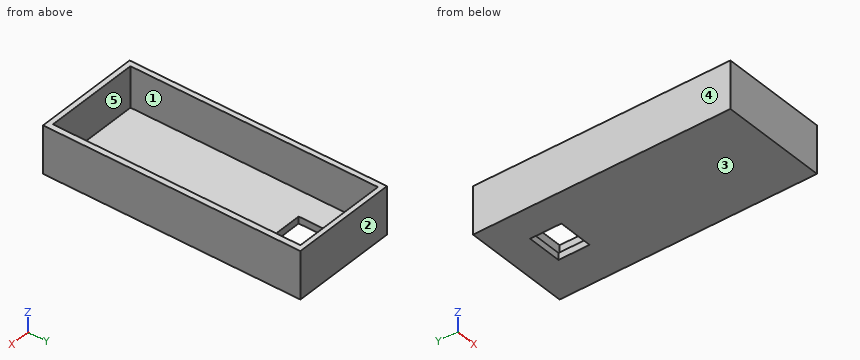
from build123d import *

# Parameters (mm, degrees)
F0_W     = 50
F0_H     = 120
F1_DEPTH = 22.1
F2_W     = 44.786031
F2_H     = 115.363243
F3_DEPTH = 18.9
F4_W     = 16.371712
F4_H     = 14.506579
F5_DEPTH = 3.2


with BuildPart() as f1:
    # F0 (on Top) → F1 (new body)
    with BuildSketch(Plane.XY):
        with Locations((25, 60)):
            Rectangle(F0_W, F0_H)
    extrude(amount=F1_DEPTH)

    # F2 (on face) → F3 (cut)
    with BuildSketch(Plane.XY.offset(22.1)):
        with Locations((24.874761, 60.085734)):
            Rectangle(F2_W, F2_H)
    extrude(amount=-F3_DEPTH, mode=Mode.SUBTRACT)

    # F4 (on face) → F5 (cut, through all)
    with BuildSketch(Plane.XY.offset(3.2)):
        with Locations((23.106907, 98.141447)):
            Rectangle(F4_W, F4_H)
    extrude(amount=-F5_DEPTH, mode=Mode.SUBTRACT)


solid = f1.part
Can you work these out from the model? Positions are in its coordinate system, mm. Face numbers are marked on the shaded views. A direction names the side the tool comes from. Round coordinates to 2 decimals unless told otherwise and drop trailing zeros. Write each loop counter-clockwise with the first axis right and the second up, starting at its lowest first coordinate (ties: lowest second). Pieces come first, ordered by that corner, then holes. Notation, with made-up numbers: M 86.5,84.25 L 144.5,84.25 A8 cw 144.5,96.25 Z; hole C 20,46.25 d11. An arc over 180 degrees is marked long. Use a Markdown table: item, result.
Item 1: Which directions (+Z, -Z, +X, -X, +Y, -Y) give clear straight access to the entire face, cutting with the end or side of a thin tool? Please do the marked faces 1 and 2.
Found:
| item | result |
|---|---|
| face 1 | +Z |
| face 2 | +Z, -Z, +X, -X, +Y |
Item 2: For pin 1 Ø2 at (x, y) = (35, 20.5) entering from +Z, with a flat end and sliding along its axis, tell me the tip position at first contact or that it passes through.
Found:
| item | result |
|---|---|
| pin 1 | stops at z = 3.2 |
Item 3: We'd pull the mould along X, two halves only. Please class the marked faces 3, 4 and 5: released by +X, released by -X, zero draft, split by the parting line, or undercut.
Found:
| item | result |
|---|---|
| face 3 | zero draft |
| face 4 | released by -X |
| face 5 | undercut |
Item 4: I want a section at C-C (y = 80). List the corners of the cut face in (x, z) for me.
Found:
| item | result |
|---|---|
| outline | M 0,0 L 50,0 L 50,22.1 L 47.27,22.1 L 47.27,3.2 L 2.48,3.2 L 2.48,22.1 L 0,22.1 Z |
Item 5: I want a section at D-D (x = 7). List the corners of the cut face in (y, z) for me, and give its area (3 significant figures).
Found:
| item | result |
|---|---|
| outline | M 0,0 L 120,0 L 120,22.1 L 117.77,22.1 L 117.77,3.2 L 2.4,3.2 L 2.4,22.1 L 0,22.1 Z |
| area | 472 mm2 |
Item 6: I want a section at A-A (x = 30). List the corners of the cut face in (y, z) for me.
Found:
| item | result |
|---|---|
| outline | M 0,0 L 90.89,0 L 90.89,3.2 L 2.4,3.2 L 2.4,22.1 L 0,22.1 Z; M 105.39,0 L 120,0 L 120,22.1 L 117.77,22.1 L 117.77,3.2 L 105.39,3.2 Z |
Item 7: I want a section at B-B (z = 15.25). List the corners of the cut face in (x, y) for me.
Found:
| item | result |
|---|---|
| outline | M 0,0 L 50,0 L 50,120 L 0,120 Z; hole M 2.48,2.4 L 47.27,2.4 L 47.27,117.77 L 2.48,117.77 Z |
Item 8: If I drill on line 1 along X through (y, z) = (18.5, 16); line 2 along Y through (x, z) = (31.5, 4.75); line 3 along Z through (x, y) = (8, 115.5), over which ranges is the centre line in solid material (lowest first)? Write a range as [from, to].
Found:
| item | result |
|---|---|
| line 1 | x = [0, 2.48], [47.27, 50] |
| line 2 | y = [0, 2.4], [117.77, 120] |
| line 3 | z = [0, 3.2] |
